Input: dimensioned drawing with shaded views. Units: mm. Origin: part minimum x, y, z. Round coordinates to 2 decimals unless told otherwise and drop trailing zeros. Loops run counter-clockwise (first coordinate to the right, second up) from the corner with the lowest first, then second, coordinate; pieces in that order, holes last.
Item 1: Ray query, L1, parallel to Z at x = 10, y = 1.35; L2, parallel to X at y = 2.7, z = 50; L3, parallel to X at y = 0.9, z = 25. Return the intervals inside material, ascending.
Item 2: Section query B-B on x = 106. Return loops of the section in (y, z).
Item 3: Section query A-A on z = 25. Return loops of the section in (x, y).
Item 4: First-contact query: P1, Ø2, axis at x = 38.5, y = 2, coming from the -Z side; P2, Ø1.2, axis at y = 2.5, z = 91, coming from the -X side; P3, Ø1.2, axis at x = 10, y = 2.5, coming from the +Z side; P4, Ø1.2, axis at y = 2, z = 6.5, coming from the +X side. Flat tips, straight axial feed; report the tip coordinate or a pass-through.
Item 5: Section query C-C on z = 65. Return loops of the section in (x, y).
Item 6: Section query D-D on y = 2.7. Give the number of separate pieces and of enclosed holes in the cut face, then the cut area to 3 significant figures.
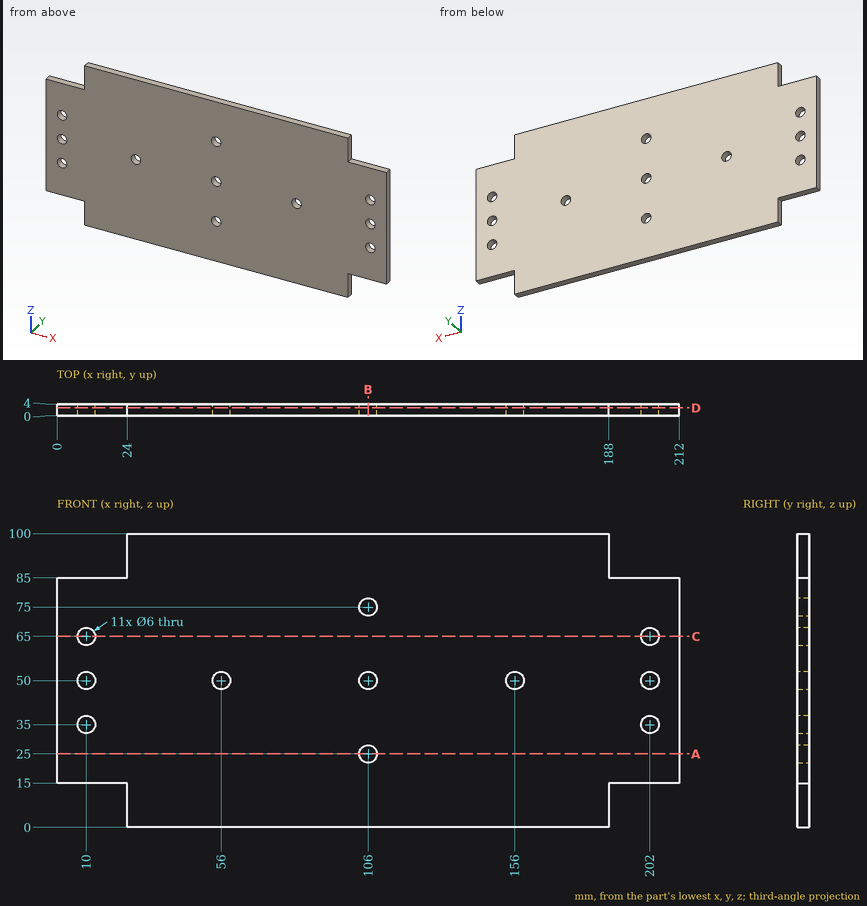
Data:
1. L1: z = 15 to 32, 38 to 47, 53 to 62, 68 to 85
1. L2: x = 0 to 7, 13 to 53, 59 to 103, 109 to 153, 159 to 199, 205 to 212
1. L3: x = 0 to 103, 109 to 212
2. outline: (0, 0) - (4, 0) - (4, 22) - (0, 22) - close; (0, 28) - (4, 28) - (4, 47) - (0, 47) - close; (0, 53) - (4, 53) - (4, 72) - (0, 72) - close; (0, 78) - (4, 78) - (4, 100) - (0, 100) - close
3. outline: (0, 0) - (103, 0) - (103, 4) - (0, 4) - close; (109, 0) - (212, 0) - (212, 4) - (109, 4) - close
4. P1: stops at z = 0
4. P2: stops at x = 24
4. P3: stops at z = 85
4. P4: stops at x = 188
5. outline: (0, 0) - (7, 0) - (7, 4) - (0, 4) - close; (13, 0) - (199, 0) - (199, 4) - (13, 4) - close; (205, 0) - (212, 0) - (212, 4) - (205, 4) - close
6. separate pieces: 1
6. enclosed holes: 11
6. area: 19,400 mm2
